```python
from build123d import *

# Parameters (mm, degrees)
SKETCH_2_R      = 4
EXTRUDE_1_DEPTH = 8
SKETCH_3_R      = 1.5
EXTRUDE_4_DEPTH = 8
RIB_1_REACH     = 70.036
SKETCH_9_WALL_W = 157.87192052
SKETCH_9_WALL_H = 8


with BuildPart() as part:
    # 草图2 → 凸台-拉伸1 (new body)
    with BuildSketch(Plane(origin=(0, 0, 0), x_dir=(1, 0, 0), z_dir=(0, 1, 0))):
        with BuildLine():
            Line((-20, 20), (-45.883337968, 9.505308716))
            ThreePointArc((-45.883337968, 9.505308716), (-52.286226701, 0), (-45.883337968, -9.505308716))
            Line((-45.883337968, -9.505308716), (-20, -20))
            Line((-20, -20), (20, -20))
            Line((20, -20), (20, 20))
            Line((20, 20), (-20, 20))
        make_face()
        with Locations(Location((-42.029303351, 0, 0), (0, 0, 270))):
            Circle(SKETCH_2_R, mode=Mode.SUBTRACT)
        with Locations(Location((-20, 9.505308716, 0), (0, 0, 270))):
            Circle(SKETCH_2_R, mode=Mode.SUBTRACT)
        with Locations(Location((-20, -9.505308716, 0), (0, 0, 270))):
            Circle(SKETCH_2_R, mode=Mode.SUBTRACT)
    extrude(amount=EXTRUDE_1_DEPTH)

    # 草图3 → 凸台-拉伸4 (add)
    with BuildSketch(Plane(origin=(20, 0, 0), x_dir=(0, 0, -1), z_dir=(1, 0, 0))):
        with BuildLine():
            Line((-20, 0), (20, 0))
            Line((20, 0), (20, 32))
            ThreePointArc((20, 32), (13.333333333, 38.666666667), (6.666666667, 32))
            ThreePointArc((6.666666667, 32), (0, 25.333333333), (-6.666666667, 32))
            ThreePointArc((-6.666666667, 32), (-13.333333333, 38.666666667), (-20, 32))
            Line((-20, 32), (-20, 0))
        make_face()
        with Locations((-13.333333333, 32)):
            Circle(SKETCH_3_R, mode=Mode.SUBTRACT)
        with Locations((13.333333333, 32)):
            Circle(SKETCH_3_R, mode=Mode.SUBTRACT)
    extrude(amount=-EXTRUDE_4_DEPTH)

    # 草图9 wall → 筋1 (add, up to next)
    with BuildSketch(Plane(origin=(5, 15, 0), x_dir=(0.707106781187, 0.707106781187, 0), z_dir=(-0.707106781187, 0.707106781187, 0)), mode=Mode.PRIVATE) as rib_1_sk1:
        Rectangle(SKETCH_9_WALL_W, SKETCH_9_WALL_H)
    rib_1_tool1 = extrude(rib_1_sk1.sketch, amount=-RIB_1_REACH, mode=Mode.PRIVATE) - part.part
    add(rib_1_tool1.solids().sort_by_distance((5, 15, 0))[0])


solid = part.part
```
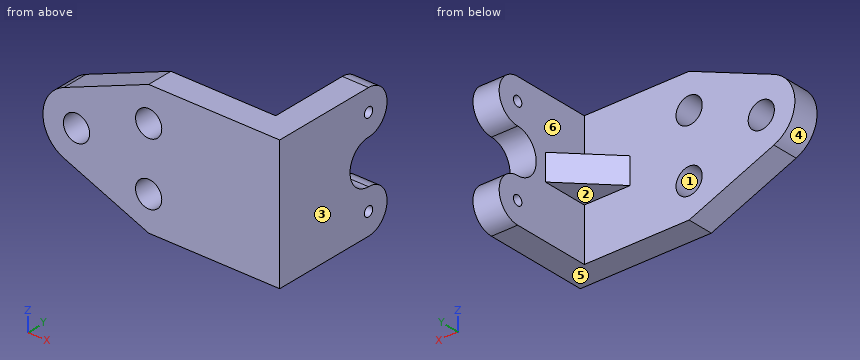
Input: part model. Units: mm. Frame: model coordinates. Face numbers are marked on the shaded views. A direction names the side the tool comes from. Round coordinates to 2 decimals unless told otherwise and drop trailing zeros. Loops run counter-clockwise (first coordinate to the right, second up) from the corner with the lowest first, then second, coordinate; pieces in that order, holes last. Notation, with made-up numbers: (-17, 85.25) - (36, 85.25) arc R32 cw to (36, 114.25) - close; hole circle Ø9 at (16.25, 19.25). An arc over 180 degrees is marked (long way). One line per item, written item: value. Start each with the question number.
(1) Section C-C, the plane y = 11. Return loops of the section in (x, z).
(2) Contact query for flat-ended pins moving along their axis: P1, Ø12, axis at x = -11.5, z = -13.5, coming from the +Y side; P2, Ø4, axis at y = 32, z = 13.33, coming from the +X side; P3, Ø7, axis at x = 7, y = 15, coming from the +Z side. Output: stop coordinate, or through.
(3) Section A-A, the plane z = 0. Return loops of the section in (x, y), plus the area to 3 significant figures.
(4) Ray query, line 1 (X direction, y = 6.5, z = 0); line 2 (X direction, y = 31.5, z = -10.5); line 3 (Y direction, x = -10, z = -4.5). Return the intervals inside material, ascending. Write a range as [from, to].
(5) Section B-B, the plane x = 1. Return loops of the section in (y, z), plus the area to 3 significant figures.
(6) Draft query along Z for the marked faces 1, 2, 3 and 4. Return one class per face: +Z half, -Z half, draft (parallel to the pull), parting line (faces both ways), or undercut.
(7) Section D-D, the plane x = -23. Return loops of the section in (y, z), plus the area to 3 significant figures.
(8) Access query for the marked faces 5 and 6. Directions: +Z, -Z, +X, -X, +Y, -Y. A direction counts if a zero-diameter tool reaches every point of the face in a straight line with its end or side. Return the directions, or none.
Results below:
1. outline: (1, -4) - (12, -4) - (12, -20) - (20, -20) - (20, 20) - (12, 20) - (12, 4) - (1, 4) - close
2. P1: y = 8
2. P2: x = 20
2. P3: z = 4
3. outline: (-52.29, 0) - (-46.03, 0) - (-46.03, 8) - (-52.29, 8) - close; (-38.03, 0) - (20, 0) - (20, 25.33) - (12, 25.33) - (12, 22) - (-2, 8) - (-38.03, 8) - close
3. area: 751 mm^2
4. line 1: [-52.29, -46.03], [-38.03, 20]
4. line 2: [12, 20]
4. line 3: [0, 8]
5. outline: (0, -20) - (8, -20) - (8, -4) - (11, -4) - (11, 4) - (8, 4) - (8, 20) - (0, 20) - close
5. area: 344 mm^2
6. face 1: undercut
6. face 2: -Z half
6. face 3: draft
6. face 4: parting line
7. outline: (0, -18.78) - (8, -18.78) - (8, -12.15) - (0, -12.15) - close; (0, -6.86) - (8, -6.86) - (8, 6.86) - (0, 6.86) - close; (0, 12.15) - (8, 12.15) - (8, 18.78) - (0, 18.78) - close
7. area: 216 mm^2
8. face 5: -Z, +X, -X, +Y, -Y
8. face 6: -X, +Y
